Read the model definition and answer for the solid it produces. Units are mm, in the model's axes. Face numbers are marked on the shaded views. A direction names the side the tool comes from. Give positions to 0.01 mm unless a question says otherwise; leave off trailing zeros. Write each loop counter-clockwise with the first axis right and the second up, starting at its lowest first coordinate (ties: lowest second). Pieces come first, ordered by that corner, then holes. Notation, with made-up numbers: M 30,80 L 53,80 A20 ccw 53,90 Z; hole C -31,54 d10. An arc over 180 degrees is marked long. Use a Markdown table: item, result. Add a question column.
Item 1: A cutting plane is placed at D-D on x = -2. Determine the outline of the cut face in (y, z).
Item 2: Given P1, Ø2, axis at x = 1.5, y = 23.5, coming from the +Z side; P2, Ø1.6, axis at x = -1, y = 33.5, coming from the -Z side, each flat-ended and moving along its own axis, determine where each tip first touches the part or whether it passes through.
Item 3: A cutting plane is placed at B-B on x = -6.5. Determine the outline of the cut face in (y, z).
Item 4: A cutting plane is placed at A-A on z = 8.5. Determine the outline of the cut face in (x, y).
Item 5: Consider probe 1 along Z at (x, y) = (-7.75, 6); probe 2 along X at (y, z) = (10, -5.5). Determine where each line is inside the solid, lowest interval first. Write a range as [from, to].
Item 6: A cutting plane is placed at C-C on z = -3.5. Determine the outline of the cut face in (x, y), then the cut area to 3 significant figures.
Item 7: For the marked faces 1, 2, 3, 4 and 5, determine the directions among +Z, -Z, +X, -X, +Y, -Y from which every point of the face is accessible in a straight line to the end or side of a thin tool.
Item 8: The mould has two halves that part along X. Classify the marked faces 6, 7 and 8: pulls with the +X half, pulls with the -X half, needs draft (parallel to the pull), parting line crosses it, or undercut.
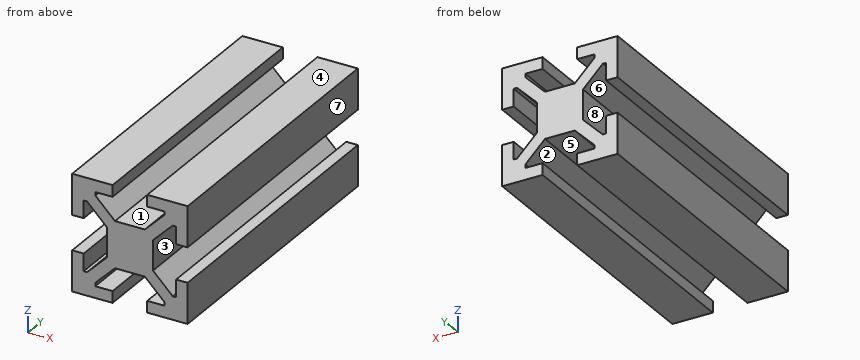
from build123d import *

# Parameters (mm, degrees)
F1_DEPTH = 50


with BuildPart() as f1:
    # F0 (on Front) → F1 (new body)
    with BuildSketch(Plane.XZ):
        Polygon((0, 0), (0, 4), (-2.585786, 4), (-6, 7.414214), (-6, 8), (-3, 8), (-3, 10), (-10, 10), (-10, 3), (-8, 3), (-8, 6), (-7.414214, 6), (-4, 2.585786), (-4, 0), align=None)
    extrude(amount=-F1_DEPTH)

    # F2: F1 across face


with BuildPart() as f1_1:
    add(f1.part)
    add(f1.part.mirror(Plane(origin=(0, 25, 2), x_dir=(0, 1, 0), z_dir=(1, 0, 0))))

    # F3: F1 across face


with BuildPart() as f1_2:
    add(f1_1.part)
    add(f1_1.part.mirror(Plane(origin=(0, 25, 0), x_dir=(1, 0, 0), z_dir=(0, 0, -1))))


solid = f1_2.part
Filled in:
| question | item | result |
|---|---|---|
| 1 | outline | M 0,-4 L 50,-4 L 50,4 L 0,4 Z |
| 2 | P1 | z = 4 |
| 2 | P2 | z = -4 |
| 3 | outline | M 0,-10 L 50,-10 L 50,-5.09 L 0,-5.09 Z; M 0,5.09 L 50,5.09 L 50,10 L 0,10 Z |
| 4 | outline | M -10,0 L -3,0 L -3,50 L -10,50 Z; M 3,0 L 10,0 L 10,50 L 3,50 Z |
| 5 | probe 1 | [-10, -6], [6, 10] |
| 5 | probe 2 | [-10, -8], [-6.91, -4.09], [4.09, 6.91], [8, 10] |
| 6 | outline | M -10,0 L -8,0 L -8,50 L -10,50 Z; M -4.91,0 L 4.91,0 L 4.91,50 L -4.91,50 Z; M 8,0 L 10,0 L 10,50 L 8,50 Z |
| 6 | area | 691 mm² |
| 7 | face 1 | +Z, +Y, -Y |
| 7 | face 2 | +Y, -Y |
| 7 | face 3 | +X, +Y, -Y |
| 7 | face 4 | +Z, +X, -X, +Y, -Y |
| 7 | face 5 | -Z, +Y, -Y |
| 8 | face 6 | undercut |
| 8 | face 7 | pulls with the +X half |
| 8 | face 8 | pulls with the -X half |
